Geometry check sheet. Reference: the model listing, model coordinates, mm. Face numbers are marked on the shaded views. A direction names the side the tool comes from. Coordinates: 2 decimals unless noted, no trailing zeros. Write each loop counter-clockwise with the first axis right and the second up, starting at its lowest first coordinate (ties: lowest second). Pieces come first, ordered by that corner, then holes.
from build123d import *


with BuildPart() as part:
    # Sketch1 → Revolve1 (revolve)
    with BuildSketch(Plane.XZ, mode=Mode.PRIVATE) as revolve1_sk:
        Polygon((6, 16.25), (6, 19), (4.92, 19), (4.92, 18.5), (3, 18.5), (3, 0.5), (4.92, 0.5), (4.92, 0), (6, 0), (6, 2.75), (5.75, 2.75), (5.75, 3.85), (6, 3.85), (6, 15.15), (5.75, 15.15), (5.75, 16.25), align=None)
    revolve(revolve1_sk.sketch.rotate(Axis((0, 0, 19), (0, 0, -1)), 180), axis=Axis((0, 0, 19), (0, 0, -1)))


solid = part.part
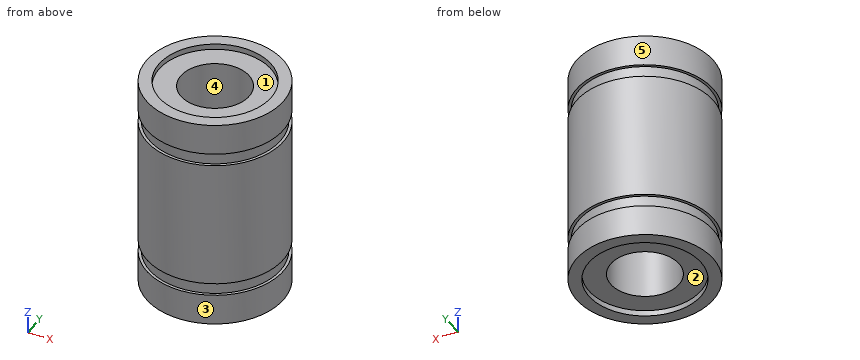
1. Thickness scan on line 1 along Z through (x, y) = (-4.25, -4); line 2 along Y through (x, z) = (0, 12.75); line 3 along Y through (x, z) = (0, 0.1). Record the ranges inside material, lowest first.
Computed values:
line 1: z = 0 to 2.75, 3.85 to 15.15, 16.25 to 19
line 2: y = -6 to -3, 3 to 6
line 3: y = -6 to -4.92, 4.92 to 6
2. Access from +Z, -Z, +X, -X, +Y, -Y to the whole of each face (thin tool, end or side, straight path). Record for the marked faces 1, 2 and 3.
Computed values:
face 1: +Z
face 2: -Z
face 3: +Z, -Z
3. Gauge pin test, flat ends, axial feed: pin 1 Ø1.5 at (x, y) = (1, -2.5) entering from +Z; pin 2 Ø1.5 at (x, y) = (-0.5, 2.5) entering from -Z; pin 3 Ø1.5 at (y, z) = (-2.5, 3.5) entering from -X. Record the tip position at first contact, or that the pin passes through.
Computed values:
pin 1: stops at z = 18.5
pin 2: stops at z = 0.5
pin 3: stops at x = -5.71
4. Sectioned sample at D-D, the plane y = -3.75. Record the boundary of the cut face in (x, z), and give its area (3 significant figures).
Computed values:
outline: (-4.68, 0) - (-3.18, 0) - (-3.18, 0.5) - (3.18, 0.5) - (3.18, 0) - (4.68, 0) - (4.68, 2.75) - (4.36, 2.75) - (4.36, 3.85) - (4.68, 3.85) - (4.68, 15.15) - (4.36, 15.15) - (4.36, 16.25) - (4.68, 16.25) - (4.68, 19) - (3.18, 19) - (3.18, 18.5) - (-3.18, 18.5) - (-3.18, 19) - (-4.68, 19) - (-4.68, 16.25) - (-4.36, 16.25) - (-4.36, 15.15) - (-4.68, 15.15) - (-4.68, 3.85) - (-4.36, 3.85) - (-4.36, 2.75) - (-4.68, 2.75) - close
area: 170 mm2
5. Draft check along X on the marked faces 4 and 5. Enter one of: released by +X, released by -X, zero draft, split by the parting line, or undercut.
Computed values:
face 4: undercut
face 5: split by the parting line
6. Sectioned sample at C-C, the plane z = 6.5. Record the boundary of the cut face in (x, y), and give its area (3 significant figures).
Computed values:
outline: circle Ø12 at (0, 0); hole circle Ø6 at (0, 0)
area: 84.8 mm2
